Verification items for the finished model (mm, model axes). Face numbers are marked on the shaded views. Round coordinates to 2 decimals unless told otherwise and drop trailing zeros. Write each loop counter-clockwise with the first axis right and the second up, starting at its lowest first coordinate (ties: lowest second). Pieces come first, ordered by that corner, then holes. Notation, with made-up numbers: (74.5, 2.25) -> (120.5, 2.25) arc R21 cw to (120.5, 25.25) -> close; hole circle Ø5 at (-12, 71.5). An arc over 180 degrees is marked (long way). Use CSV: the item, a comma, the result in double quotes.
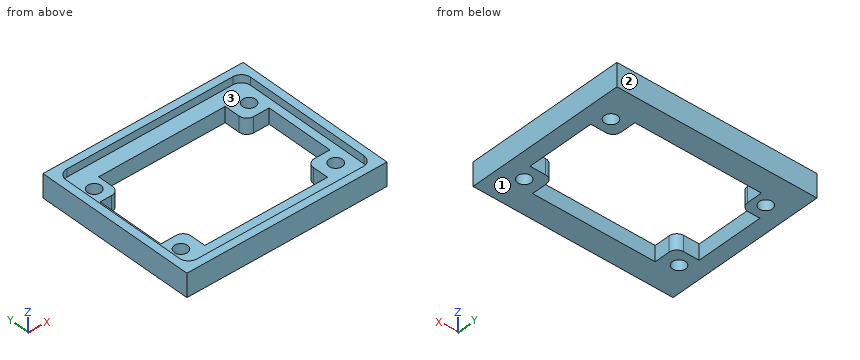
Autodesk Inventor part; units mm, degrees
ref_plane "YZ Plane" through (0, 0, 0) normal (1, 0, 0) x (0, 1, 0)
ref_plane "XZ Plane" through (0, 0, 0) normal (0, 1, 0) x (-1, 0, 0)
ref_plane "XY Plane" through (0, 0, 0) normal (0, 0, 1) x (1, 0, 0)
sketch "Эскиз1" plane through (0, 0, 0) normal (0, 0, 1) x (1, 0, 0)
  line L0 (0, 0) -> (47.7, 0)
  line L1 (47.7, 0) -> (47.7, 37.5)
  line L2 (47.7, 37.5) -> (0, 37.5)
  line L3 (0, 37.5) -> (0, 0)
  line L4 (3.85, 31.25) -> (43.85, 31.25) construction
  line L5 (43.85, 31.25) -> (43.85, 6.25) construction
  line L6 (43.85, 6.25) -> (3.85, 6.25) construction
  line L7 (3.85, 6.25) -> (3.85, 31.25) construction
  line L8 (3.85, 31.25) -> (3.85, 37.5) construction
  line L9 (3.85, 6.25) -> (3.85, 0) construction
  line L10 (3.85, 31.25) -> (0, 31.25) construction
  line L11 (43.85, 31.25) -> (47.7, 31.25) construction
  circle A0 centre (3.85, 31.25) radius 1.7
  circle A1 centre (43.85, 31.25) radius 1.7
  circle A2 centre (43.85, 6.25) radius 1.7
  circle A3 centre (3.85, 6.25) radius 1.7
  dimension "d0" = 47.7
  dimension "d1" = 37.5
  dimension "d2" = 40
  dimension "d3" = 25
  dimension "d6" = 3.4
extrude "Выдавливание1" add sketch "Эскиз1" along normal blind 4
sketch "Эскиз2" plane through (0, 0, 4) normal (0, 0, 1) x (1, 0, 0)
  circle A0 centre (3.85, 6.25) radius 1.7
  circle A1 centre (43.85, 6.25) radius 1.7
  circle A2 centre (43.85, 31.25) radius 1.7
  circle A3 centre (3.85, 31.25) radius 1.7
  line L0 (0, 0) -> (47.7, 0)
  line L1 (47.7, 0) -> (47.7, 37.5)
  line L2 (47.7, 37.5) -> (0, 37.5)
  line L3 (0, 37.5) -> (0, 0)
  line L4 (-2, 39.5) -> (49.7, 39.5)
  line L5 (49.7, 39.5) -> (49.7, -2)
  line L6 (49.7, -2) -> (-2, -2)
  line L7 (-2, -2) -> (-2, 39.5)
  dimension "d9" = 2
extrude "Выдавливание2" add sketch "Эскиз2" along normal blind 2 and the other way blind 4 contours L4 L5 L6 L7
fillet "Сопряжение1" radius 2.4 4 edges at (0, 37.5, 5) (47.7, 37.5, 5) (47.7, 0, 5) (0, 0, 5)
sketch "Эскиз3" plane through (0, 0, 4) normal (0, 0, 1) x (1, 0, 0)
  line L0 (7, 33.5) -> (39.7, 33.5)
  line L1 (39.7, 4) -> (8, 4)
  line L2 (2.4, 37.5) -> (45.3, 37.5)
  line L3 (47.7, 35.1) -> (47.7, 2.4)
  line L4 (2, 27.5) -> (7, 27.5)
  line L5 (8, 10) -> (2, 10)
  line L6 (2, 10) -> (2, 27.5)
  line L7 (39.7, 27.5) -> (45.7, 27.5)
  line L8 (45.7, 27.5) -> (45.7, 10)
  line L9 (45.7, 10) -> (39.7, 10)
  line L10 (45.3, 0) -> (2.4, 0)
  line L11 (0, 2.4) -> (0, 35.1)
  line L12 (8, 4) -> (8, 10)
  line L13 (7, 27.5) -> (7, 33.5)
  line L14 (39.7, 33.5) -> (39.7, 27.5)
  line L15 (39.7, 10) -> (39.7, 4)
  point P0 (0, 0)
  dimension "d15" = 4
  dimension "d17" = 4
  dimension "d24" = 10
  dimension "d25" = 10
  dimension "d26" = 10
  dimension "d27" = 10
  dimension "d28" = 2
  dimension "d29" = 2
  dimension "d33" = 8
  dimension "d34" = 7
  dimension "d35" = 8
  dimension "d36" = 8
extrude "Выдавливание3" cut sketch "Эскиз3" against normal blind 10
fillet "Сопряжение2" radius 2 4 edges at (8, 10, 2) (7, 27.5, 2) (39.7, 27.5, 2) (39.7, 10, 2)
properties part number "forpower"
Q1. Mould release check, pull along Y, two halves, no side actions. Record for the marked faces 1, 2 and 3: released by +Y, released by -Y, zero draft, split by the parting line, or undercut.
Filled in:
face 1,"zero draft"
face 2,"released by +Y"
face 3,"undercut"
Q2. Section check B-B (z = 5.2). Record the cut outline in (x, y).
Filled in:
outline,"(-2, -2) -> (49.7, -2) -> (49.7, 39.5) -> (-2, 39.5) -> close; hole (0, 2.4) arc R2.4 ccw to (2.4, 0) -> (45.3, 0) arc R2.4 ccw to (47.7, 2.4) -> (47.7, 35.1) arc R2.4 ccw to (45.3, 37.5) -> (2.4, 37.5) arc R2.4 ccw to (0, 35.1) -> close"
Q3. Section check C-C (x = 17.5). Record the cut outline in (y, z), plus the area to 3 significant figures.
Filled in:
outline,"(-2, 0) -> (4, 0) -> (4, 4) -> (0, 4) -> (0, 6) -> (-2, 6) -> close; (33.5, 0) -> (39.5, 0) -> (39.5, 6) -> (37.5, 6) -> (37.5, 4) -> (33.5, 4) -> close"
area,"56.0 mm²"
Q4. Section check A-A (y = 6.25). Record the cut outline in (x, z).
Filled in:
outline,"(-2, 0) -> (2.15, 0) -> (2.15, 4) -> (0, 4) -> (0, 6) -> (-2, 6) -> close; (5.55, 0) -> (8, 0) -> (8, 4) -> (5.55, 4) -> close; (39.7, 0) -> (42.15, 0) -> (42.15, 4) -> (39.7, 4) -> close; (45.55, 0) -> (49.7, 0) -> (49.7, 6) -> (47.7, 6) -> (47.7, 4) -> (45.55, 4) -> close"
Q5. Go/stop test with flat-tipped pins: P1, Ø2.5, axis at x = 3.85, y = 31.25, coming from the +Z side; P2, Ø3, axis at x = 32, y = 32.5, coming from the +Z side. Record where each tip stops, or that it passes through.
Filled in:
P1,"through"
P2,"z = 4"
Q6. Section check D-D (y = 21). Record the cut outline in (x, z).
Filled in:
outline,"(-2, 0) -> (2, 0) -> (2, 4) -> (0, 4) -> (0, 6) -> (-2, 6) -> close; (45.7, 0) -> (49.7, 0) -> (49.7, 6) -> (47.7, 6) -> (47.7, 4) -> (45.7, 4) -> close"
Q7. Material ranges on L1, parallel to Y at x = 3.85, z = 3.25; L2, parallel to Y at x = 27, z = 2.8; L3, parallel to X at y = 34, z = 5.5, recorded low to high.
Filled in:
L1,"-2 to 4.55, 7.95 to 10, 27.5 to 29.55, 32.95 to 39.5"
L2,"-2 to 4, 33.5 to 39.5"
L3,"-2 to 0, 47.7 to 49.7"
